Check sheet for the modelled part. Datum: model origin and axes. Units: mm. Coordinates: 2 decimals unless noted, no trailing zeros. Loops run counter-clockwise (first coordinate to the right, second up) from the corner with the lowest first, then second, coordinate; pieces in that order, holes last.
```python
from build123d import *

# Parameters (mm, degrees)
F0_W     = 254
F0_H     = 254
F1_DEPTH = 254
F2_R     = 95.25
F3_DEPTH = 254.001
F4_SIZE  = 25.4


with BuildPart() as f1:
    # F0 (on Top) → F1 (new body)
    with BuildSketch(Plane.XY):
        with Locations((127, -127)):
            Rectangle(F0_W, F0_H)
    extrude(amount=F1_DEPTH)

    # F2 (on face) → F3 (cut, through all)
    with BuildSketch(Plane.XY.offset(254)):
        with Locations((127, -127)):
            Circle(F2_R)
    extrude(amount=-F3_DEPTH, mode=Mode.SUBTRACT)

    # F4
    f4_edges = [f1.edges().sort_by_distance(p)[0] for p in [
        (127, -254, 254),
        (254, -127, 254),
        (127, 0, 254),
        (0, -127, 254),
        (254, -127, 0),
        (127, -254, 0),
        (127, 0, 0),
        (0, -127, 0),
    ]]
    chamfer(f4_edges, length=F4_SIZE)


solid = f1.part
```
1) Mould release check, pull along Y, two halves, no side actions. Record for faces 1 (the flat face through (96, -36, 0)), 2 (the cylindrical face through (170.952, -211.503, 128.778)), 3 (the flat face through (125, -254, 126)): +Y half, -Y half, draft (parallel to the pull), parting line (faces both ways), or undercut.
Answer sheet:
face 1: draft
face 2: undercut
face 3: -Y half
2) Section check B-B on x = 127. Enter the section's corners in (y, z).
Answer sheet:
outline: (-254, 25.4) - (-228.6, 0) - (-222.25, 0) - (-222.25, 254) - (-228.6, 254) - (-254, 228.6) - close; (-31.75, 0) - (-25.4, 0) - (0, 25.4) - (0, 228.6) - (-25.4, 254) - (-31.75, 254) - close
3) Section check A-A on y = -127. Enter the section's corners in (x, z).
Answer sheet:
outline: (0, 25.4) - (25.4, 0) - (31.75, 0) - (31.75, 254) - (25.4, 254) - (0, 228.6) - close; (222.25, 0) - (228.6, 0) - (254, 25.4) - (254, 228.6) - (228.6, 254) - (222.25, 254) - close
4) Scan lines: line 1 (Y direction, x = 127, z = 88); line 2 (Y direction, x = 213, z = 152.5); line 3 (X direction, y = -84, z = 82.5). Record each from-to range of solid material in increasing order.
Answer sheet:
line 1: y = -254 to -222.25, -31.75 to 0
line 2: y = -254 to -167.95, -86.05 to 0
line 3: x = 0 to 42.01, 211.99 to 254
5) Section check D-D on z = 142. Enter the section's corners in (x, y).
Answer sheet:
outline: (0, -254) - (254, -254) - (254, 0) - (0, 0) - close; hole circle Ø190.5 at (127, -127)
6) Section check C-C on y = -238. Enter the section's corners in (x, z), plus the area to 3 significant figures.
Answer sheet:
outline: (0, 25.4) - (16, 9.4) - (238, 9.4) - (254, 25.4) - (254, 228.6) - (238, 244.6) - (16, 244.6) - (0, 228.6) - close
area: 59,200 mm2
